Verification items for the finished model (mm, model axes). A direction names the side the tool comes from. Give positions to 0.01 mm unless a question says otherwise; leave off trailing zeros. Order: outer loops, then holes, each group sorted by start corner. A loop starts at its lowest first (then second) coordinate and runs counter-clockwise, first axis right, second up.
from build123d import *

# Parameters (mm, degrees)
F0_R     = 25
F1_DEPTH = 20
F2_SIZE  = 5
F3_SIZE  = 5
F4_R     = 15
F5_DEPTH = 5
F6_R     = 15
F7_DEPTH = 5
F8_R     = 6.5
F8_R_2   = 5
F9_DEPTH = 20
F10_T    = 2.5


# Not quite as in the source:
# - a shell that OpenCascade refuses in one call is made with other operations: the cavity is built on its own and cut out


with BuildPart() as f1:
    # F0 (on Right) → F1 (new body)
    with BuildSketch(Plane.YZ):
        Circle(F0_R)
    extrude(amount=F1_DEPTH)

    # F2
    f2_edges = [f1.edges().sort_by_distance(p)[0] for p in [
        (20, -25, 0),
    ]]
    chamfer(f2_edges, length=F2_SIZE)

    # F3
    f3_edges = [f1.edges().sort_by_distance(p)[0] for p in [
        (0, -25, 0),
    ]]
    chamfer(f3_edges, length=F3_SIZE)

    # F4 (on face) → F5 (cut)
    with BuildSketch(Plane(origin=(0, 0, 0), x_dir=(0, -1, 0), z_dir=(-1, 0, 0))):
        Circle(F4_R)
    extrude(amount=-F5_DEPTH, mode=Mode.SUBTRACT)

    # F6 (on face) → F7 (cut)
    with BuildSketch(Plane.YZ.offset(20)):
        Circle(F6_R)
    extrude(amount=-F7_DEPTH, mode=Mode.SUBTRACT)

    # F8 (on face) → F9 (join)
    with BuildSketch(Plane(origin=(5, 0, 0), x_dir=(0, -1, 0), z_dir=(-1, 0, 0))):
        Circle(F8_R)
        Circle(F8_R_2, mode=Mode.SUBTRACT)
    extrude(amount=F9_DEPTH)

    # F10: shell of thickness 2.5, made by hand


with BuildPart() as f10_core1:
    # F10_t2: copy of F1
    add(f1.part)

    # the walls: a layer under each face that stays
    f10_faces = [f10_core1.faces().sort_by_distance(p)[0] for p in [
        (10, -25, 0),
        (2.5, -22.5, 0),
        (17.5, -22.5, 0),
        (0, -13.3333333333, -13.3333333333),
        (20, -13.3333333333, -13.3333333333),
        (2.5, 15, 0),
        (17.5, -15, 0),
        (5, 10, -10),
        (15, 0, 0),
        (-5, 6.5, 0),
        (-5, 5, 0),
        (5, 0, 0),
    ]]
    thicken(f10_faces, amount=-F10_T, mode=Mode.SUBTRACT)

    # F10_s3 → F10_t4 (revolve, cut)
    with BuildSketch(Plane.XY):
        Polygon((4.975, -14.975), (5, -17.5), (7.5, -17.5), (7.5, -15), align=None)
    revolve(axis=Axis((5, 0, 0), (-1, 0, 0)), mode=Mode.SUBTRACT)

    # F10_s5 → F10_t6 (revolve, cut)
    with BuildSketch(Plane.XY):
        Polygon((15.025, 14.975), (15, 17.5), (12.5, 17.5), (12.5, 15), align=None)
    revolve(axis=Axis((15, 0, 0), (1, 0, 0)), mode=Mode.SUBTRACT)

    # F10_s7 → F10_t8 (revolve, cut)
    with BuildSketch(Plane.XY):
        Polygon((4.975, -6.525), (7.5, -6.5), (7.5, -4), (5, -4), align=None)
    revolve(axis=Axis((5, 0, 0), (-1, 0, 0)), mode=Mode.SUBTRACT)

    # F10_s9 → F10_t10 (revolve, cut)
    with BuildSketch(Plane.XY):
        Polygon((4.975, -4.975), (5, -7.5), (7.5, -7.5), (7.5, -5), align=None)
    revolve(axis=Axis((5, 0, 0), (-1, 0, 0)), mode=Mode.SUBTRACT)


with BuildPart() as f1_1:
    add(f1.part)

    # what is left inside the walls is the cavity
    f10_cavity = [f10_core1.part.solids().sort_by_distance(p)[0] for p in [
        (11.321489, -22.475, 0),
    ]]
    add(f10_cavity, mode=Mode.SUBTRACT)


solid = f1_1.part
(1) Section check A-A, the plane x = 3.5. Enter the section's corners in (y, z), then the cut area to 3 significant figures.
Solved:
outline: circle Ø47 at (0, 0); circle Ø35 at (0, 0); circle Ø13 at (0, 0); hole circle Ø39.93 at (0, 0); hole circle Ø30 at (0, 0); hole circle Ø10 at (0, 0)
area: 792 mm2
(2) Release check for a two-part mould opening along X. For faces 1 (the flat face through (5, -3, -6)), 2 (the cylindrical face through (15.035, -13.887, -10.648)), 3 (the cylindrical face through (9.944, 10.382, -19.961)), 4 (the conical face through (19.76, -16.06, -12.32)) record: pulls with the +X half, pulls with the -X half, needs draft (parallel to the pull), parting line crosses it, or undercut.
Solved:
face 1: pulls with the -X half
face 2: undercut
face 3: undercut
face 4: pulls with the +X half
(3) Section check C-C, the plane x = -10.5. Enter the section's corners in (y, z), then the cut area to 3 significant figures.
Solved:
outline: circle Ø13 at (0, 0); hole circle Ø10 at (0, 0)
area: 54.2 mm2
(4) Go/stop test with flat-tipped pins: pin 1 (12 mm diameter, centred on y = 20, z = 11.5, fed in from -X); pin 2 (12 mm diameter, centred on x = 14.5, y = -8, fed in from +Z); pin 3 (5 mm diameter, centred on y = -1, z = 1.5, fed in from -X). Record where each tip stops, or that it passes through.
Solved:
pin 1: stops at x = 0
pin 2: stops at z = 24.92
pin 3: stops at x = 5
(5) Scan lines: line 1 (X direction, y = 10, z = -3.5); line 2 (X direction, y = -4, z = 16); line 3 (Z direction, x = 16.25, y = 0). Record each from-to range of solid material in increasing order.
Solved:
line 1: x = 5 to 7.5, 12.5 to 15
line 2: x = 0 to 7.5, 12.5 to 20
line 3: z = -23.75 to -20.21, -17.5 to -15, 15 to 17.5, 20.21 to 23.75
(6) Set-up check for faces 5 (the flat face through (15, 0, 0)), 6 (the flat face through (2.5, 6, -17)), 7 (the cylindrical face through (-4.86, 5.158, -3.955)): record each of +Z, -Z, +X, -X, +Y, -Y from which the full face is reachable in a straight line by a thin tool's end or side.
Solved:
face 5: +X
face 6: none
face 7: -X
(7) Section check B-B, the plane x = 9.5. Enter the section's corners in (y, z), then the cut area to 3 significant figures.
Solved:
outline: circle Ø50 at (0, 0); hole circle Ø45 at (0, 0)
area: 373 mm2
